Source: CAD feature listing. Evaluate the final solid. Frame: model axes, mm. Round coordinates to 2 decimals unless told otherwise and drop trailing zeros. Loops run counter-clockwise (first coordinate to the right, second up) from the corner with the lowest first, then second, coordinate; pieces in that order, holes last. Notation, with made-up numbers: (-5, -10) -> (22, -10) arc R19 ccw to (22, 5) -> close; hole circle Ø2 at (14, 5). An arc over 180 degrees is marked (long way). Put each result on its own line as item: value. Start each with the question number.
1. Cut plane A-A (z = -19). Return the cut outline in (x, y), then the cut area to 3 significant figures.
2. Cut plane B-B (x = 8). Return the cut outline in (y, z).
3. Contact query for flat-ended pins moving along their axis: pin 1 (1.2 mm diameter, centred on x = -30.5, z = 5.5, fed in from +Y); pin 2 (12 mm diameter, centred on x = 21.5, z = 26.5, fed in from +Y). Output: stop coordinate, or through.
4. Cut plane C-C (y = 4). Return the cut outline in (x, z), then the cut area to 3 significant figures.
5. Material intervals for L1, parallel to Z at x = -18.5, y = 7; L2, parallel to X at y = 1.25, z = 20.5; L3, parallel to X at y = 6.5, z = 4, sorted ascending.
```python
from build123d import *

# Parameters (mm, degrees)
SKETCH1_W             = 75.4
SKETCH1_H             = 75.4
BASE_DEPTH            = 7.5
SKETCH2_W             = 66.2
SKETCH2_H             = 60.2
SLOT_DEPTH            = 1.6
SKETCH3_W             = 58.357887306
SKETCH3_H             = 60.2
SLOT_COMPONENTS_DEPTH = 5.9
FILLET2_R             = 10


with BuildPart() as part:
    # Sketch1 → Base (new body)
    with BuildSketch(Plane(origin=(0, 0, 0), x_dir=(1, 0, 0), z_dir=(0, 1, 0))):
        Rectangle(SKETCH1_W, SKETCH1_H)
    extrude(amount=BASE_DEPTH)

    # Sketch2 → Slot (cut)
    with BuildSketch(Plane(origin=(0, 7.5, 0), x_dir=(1, 0, 0), z_dir=(0, 1, 0))):
        Rectangle(SKETCH2_W, SKETCH2_H)
    extrude(amount=-SLOT_DEPTH, mode=Mode.SUBTRACT)

    # Sketch3 → Slot-Components (cut)
    with BuildSketch(Plane(origin=(0, 5.9, 0), x_dir=(1, 0, 0), z_dir=(0, 1, 0))):
        Rectangle(SKETCH3_W, SKETCH3_H)
    extrude(amount=-SLOT_COMPONENTS_DEPTH, mode=Mode.SUBTRACT)

    # Fillet2
    fillet2_edges = [part.edges().sort_by_distance(p)[0] for p in [
        (37.7, 3.75, 37.7),
        (-37.7, 3.75, 37.7),
        (-37.7, 3.75, -37.7),
        (37.7, 3.75, -37.7),
    ]]
    fillet(fillet2_edges, radius=FILLET2_R)


solid = part.part
```
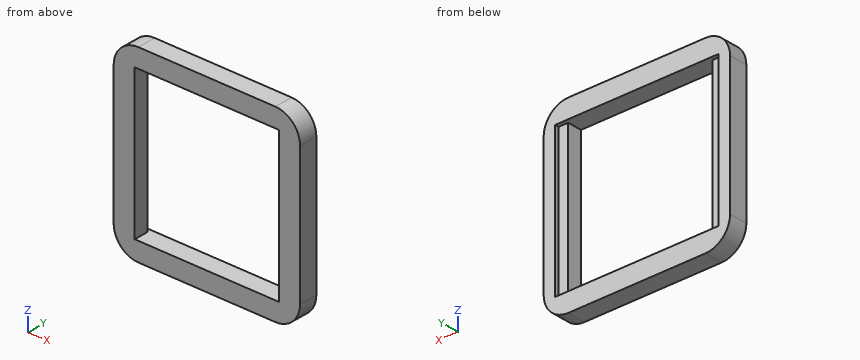
Solution:
1. outline: (-37.7, 0) -> (-29.18, 0) -> (-29.18, 5.9) -> (-33.1, 5.9) -> (-33.1, 7.5) -> (-37.7, 7.5) -> close; (29.18, 0) -> (37.7, 0) -> (37.7, 7.5) -> (33.1, 7.5) -> (33.1, 5.9) -> (29.18, 5.9) -> close
1. area: 115 mm^2
2. outline: (0, -37.7) -> (7.5, -37.7) -> (7.5, -30.1) -> (0, -30.1) -> close; (0, 30.1) -> (7.5, 30.1) -> (7.5, 37.7) -> (0, 37.7) -> close
3. pin 1: stops at y = 5.9
3. pin 2: stops at y = 7.5
4. outline: (-37.7, -27.7) arc R10 ccw to (-27.7, -37.7) -> (27.7, -37.7) arc R10 ccw to (37.7, -27.7) -> (37.7, 27.7) arc R10 ccw to (27.7, 37.7) -> (-27.7, 37.7) arc R10 ccw to (-37.7, 27.7) -> close; hole (-29.18, -30.1) -> (29.18, -30.1) -> (29.18, 30.1) -> (-29.18, 30.1) -> close
4. area: 2,090 mm^2
5. L1: z = -37.7 to -30.1, 30.1 to 37.7
5. L2: x = -37.7 to -29.18, 29.18 to 37.7
5. L3: x = -37.7 to -33.1, 33.1 to 37.7
